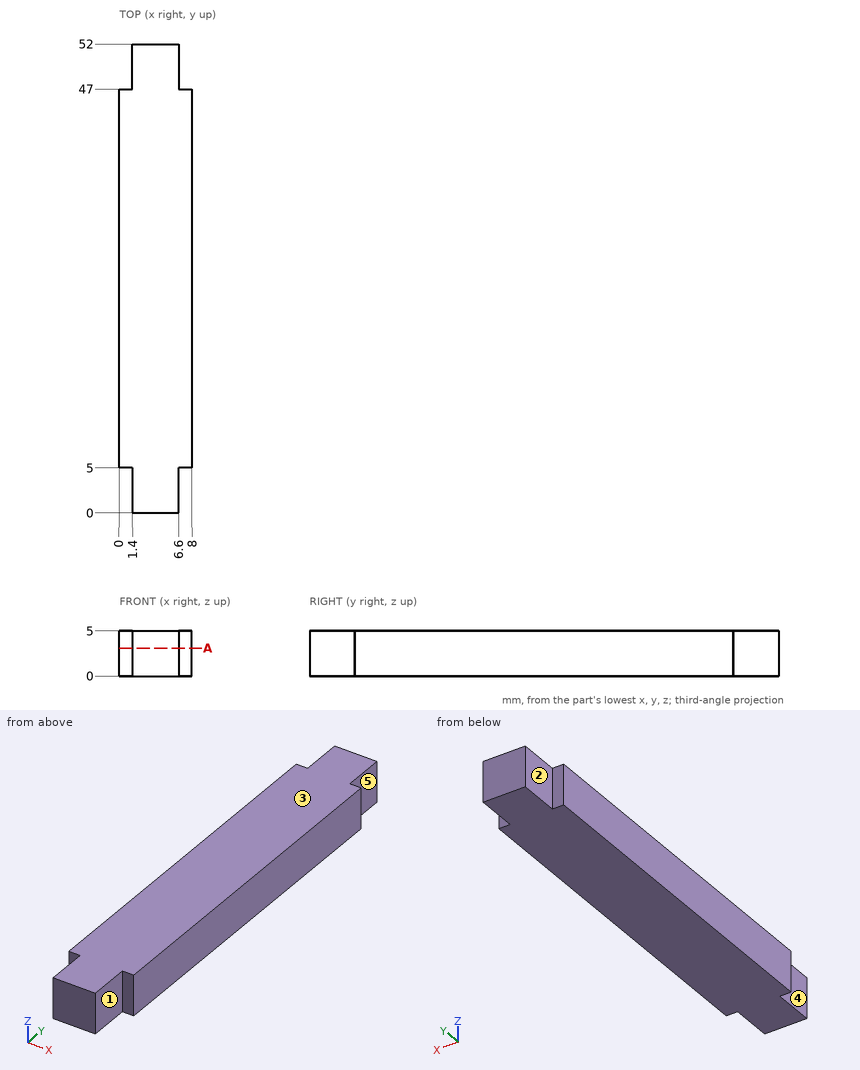
The figure shows three views and two pictorial views of one solid part (mm, origin at its lowest corner). Answer the questions. A direction names the side the tool comes from. Round coordinates to 2 decimals unless told otherwise and drop trailing zeros. Loops run counter-clockwise (first coordinate to the right, second up) from the corner with the lowest first, then second, coordinate; pieces in that order, holes last. Notation, with made-up numbers: M -18.5,52.25 L 9.5,52.25 A34 ccw 9.5,86.25 Z; hole C 43,28.25 d10. An arc over 180 degrees is marked long. Write each question's results on one line, items separated by ' | '. Start each with the question number.
1) Which of the six approach directions +Z, -Z, +X, -X, +Y, -Y give full straight-line access (tool end or side, diameter ignored) to the marked faces 1, 2, 3, 4 and 5?
2) Find section A-A on z = 3.1. Write down the section's boundary in (x, y).
3) Straight lines are drawn through the part: probe 1 along X at (y, z) = (47.5, 4.1); probe 2 along Y at (x, z) = (7.5, 1.8). For each, find the intervals that lie inside material, in ascending order.
4) Each of these flat-tipped pins is pushed along its axis until it touches: pin 1 (1.1 mm diameter, centred on x = 0.5, z = 2.5, fed in from +Y); pin 2 (1.5 mm diameter, centred on y = 50.5, z = 2, fed in from +X). Where does it stop, or does it pass through?
Final values:
1) face 1: +Z, -Z, +X, -Y | face 2: +Z, -Z, -X, +Y | face 3: +Z, +X, -X, +Y, -Y | face 4: +Z, -Z, -X, -Y | face 5: +Z, -Z, +X, +Y
2) outline: M 0,5 L 1.4,5 L 1.4,0 L 6.6,0 L 6.6,5 L 8,5 L 8,47 L 6.6,47 L 6.6,52 L 1.4,52 L 1.4,47 L 0,47 Z
3) probe 1: 1.4 to 6.6 | probe 2: 5 to 47
4) pin 1: y = 47 | pin 2: x = 6.6
